Part model, mm, in its own coordinate system. A direction names the side the tool comes from. Give positions to 0.01 mm unless a question says otherwise; leave off trailing zeros. Order: outer loops, then holes, each group sorted by start corner. A loop starts at its lowest first (then second) coordinate and runs counter-clockwise, first axis right, second up. Notation, with made-up numbers: M 14.5,48 L 46.5,48 A33 ccw 46.5,80 Z; hole C 0.25,-4 d5. An arc over 180 degrees is marked long. Return JSON: item names as keys, results as strings.
from build123d import *

# Parameters (mm, degrees)
F1_DEPTH      = 10
F2_R          = 8
F3_T          = -1.5
F4_W          = 14.2378706528
F4_H          = 10
F5_DEPTH      = 50
F7_W          = 14.2378706528
F7_H          = 10
F8_DEPTH      = 50
F6_W          = 14.2378706528
F6_H          = 10
F9_DEPTH      = 50
F10_T         = 1.5
F10_T3_DEPTH  = 13
F10_T5_DEPTH  = 17.2378706528
F10_T7_DEPTH  = 17.2378706528
F10_T10_ANGLE = 72.000000001
F10_T12_ANGLE = 72.000000001
F10_T14_ANGLE = 72.000000001
F10_T16_ANGLE = 72.000000001
F10_T18_ANGLE = 72.000000001


# Not quite as in the source:
# - a shell that OpenCascade refuses in one call is made with other operations: the cavity is built on its own and cut out


with BuildPart() as f1:
    # F0 (on Top) → F1 (new body)
    with BuildSketch(Plane.XY):
        Polygon((20.9232433585, 6.7983738762), (0, 22), (-20.9232433585, 6.7983738762), (-12.9312755504, -17.7983738762), (12.9312755504, -17.7983738762), align=None)
    extrude(amount=F1_DEPTH)

    # F2
    f2_edges = [f1.edges().sort_by_distance(p)[0] for p in [
        (20.923243, 6.798374, 5),
        (0, 22, 5),
        (12.931276, -17.798374, 5),
        (-12.931276, -17.798374, 5),
        (-20.923243, 6.798374, 5),
    ]]
    fillet(f2_edges, radius=F2_R)

    # F3
    f3_openings = [f1.faces().sort_by_distance(p)[0] for p in [
        (0, 0, 0),
    ]]
    offset(amount=F3_T, openings=f3_openings)

    # F4 (on face) → F5 (join)
    with BuildSketch(Plane(origin=(16.9272594545, -5.5, 0), x_dir=(0.3090169944, 0.9510565163, 0), z_dir=(0.9510565163, -0.3090169944, 0))):
        with Locations((0, 5)):
            Rectangle(F4_W, F4_H)
    extrude(amount=F5_DEPTH)

    # F7 (on face) → F8 (join)
    with BuildSketch(Plane(origin=(10.4616216792, 14.3991869381, 0), x_dir=(-0.8090169944, 0.5877852523, 0), z_dir=(0.5877852523, 0.8090169944, 0))):
        with Locations((0, 5)):
            Rectangle(F7_W, F7_H)
    extrude(amount=F8_DEPTH)

    # F6 (on face) → F9 (join)
    with BuildSketch(Plane(origin=(-16.9272594545, -5.5, 0), x_dir=(0.3090169944, -0.9510565163, 0), z_dir=(-0.9510565163, -0.3090169944, 0))):
        with Locations((0, 5)):
            Rectangle(F6_W, F6_H)
    extrude(amount=F9_DEPTH)

    # F10: shell of thickness 1.5, made by hand


with BuildPart() as f10_core1:
    # F10_t2: copy of F1
    add(f1.part)

    # the walls: a layer under each face that stays
    f10_faces = [f10_core1.faces().sort_by_distance(p)[0] for p in [
        (0, 20.11145618, 5),
        (-10.4616216792, 14.3991869381, 5),
        (-19.1271314522, 6.2147817412, 5),
        (-11.8212173447, -16.2705098312, 5),
        (0, -17.7983738762, 5),
        (11.8212173447, -16.2705098312, 5),
        (38.5038003641, -19.9959346906, 5),
        (42.9035443596, -6.4549150281, 5),
        (19.1271314522, 6.2147817412, 5),
        (30.9155926475, 30.4402066006, 5),
        (19.3969133257, 38.8090169944, 5),
        (17.7005466777, 5.7512562497, 4.25),
        (10.9395394663, -15.0569843397, 4.25),
        (0, -16.2983738762, 4.25),
        (-10.9395394663, -15.0569843397, 4.25),
        (-17.7005466777, 5.7512562497, 4.25),
        (-9.5799438008, 13.1856614466, 4.25),
        (0, 18.61145618, 4.25),
        (0, 15.6565411519, 10),
        (-42.9035443596, -6.4549150281, 5),
        (-38.5038003641, -19.9959346906, 5),
        (0, 1.1565411519, 8.5),
    ]]
    thicken(f10_faces, amount=-F10_T, mode=Mode.SUBTRACT)

    # F10_s4 → F10_t3 (cut)
    with BuildSketch(Plane.XY.offset(-1.5)):
        Polygon((4.6989635422, 18.6045441687), (3.8206041399, 17.3700666434), (5.0341296315, 16.488388765), (5.9158075099, 17.7019142566), align=None)
        Polygon((-19.1460325548, 1.2801404241), (-17.7005466777, 1.7340353228), (-17.2370211862, 0.3074505484), (-18.6636059606, -0.1560749432), align=None)
        Polygon((-14.7370180496, -12.2894109339), (-13.3008026823, -11.8069843397), (-13.7643281739, -10.3803995652), (-15.1909129483, -10.8439250568), align=None)
        Polygon((14.7370180496, -12.2894109339), (13.3008026823, -11.8069843397), (13.7643281739, -10.3803995652), (15.1909129483, -10.8439250568), align=None)
        Polygon((19.1460325548, 1.2801404241), (18.6636059606, -0.1560749432), (17.2370211862, 0.3074505484), (17.7005466777, 1.7340353228), align=None)
        Polygon((16.2419133739, 10.2181002174), (15.3392834617, 9.0012562497), (14.1257579702, 9.8829341281), (15.0074358486, 11.0964596197), align=None)
    extrude(amount=F10_T3_DEPTH, mode=Mode.SUBTRACT)

    # F10_s6 → F10_t5 (cut)
    with BuildSketch(Plane.YZ.offset(-8.6189353264)):
        Polygon((-16.2833738762, 8.485), (-17.7983738762, 8.5), (-17.7983738762, 10), (-16.2983738762, 10), align=None)
    extrude(amount=F10_T5_DEPTH, mode=Mode.SUBTRACT)

    # F10_s8 → F10_t7 (cut)
    with BuildSketch(Plane(origin=(6.9728651525, 5.0660830753, 0), x_dir=(0, 0, 1), z_dir=(-0.8090169944, -0.5877852523, 0))):
        Polygon((8.485, 16.2833738762), (8.5, 17.7983738762), (10, 17.7983738762), (10, 16.2983738762), align=None)
    extrude(amount=F10_T7_DEPTH, mode=Mode.SUBTRACT)

    # F10_s9 → F10_t10 (revolve, cut)
    with BuildSketch(Plane(origin=(2.1998719977, 6.7705098312, 0), x_dir=(0, 0, 1), z_dir=(-0.3090169944, -0.9510565163, 0))):
        Polygon((8.485, -16.2833738762), (8.5, -17.7983738762), (10, -17.7983738762), (10, -16.2983738762), align=None)
    revolve(axis=Axis((11.5186793218, 3.7426457862, 8.5), (0, 0, 1)), revolution_arc=F10_T10_ANGLE, mode=Mode.SUBTRACT)

    # F10_s11 → F10_t12 (revolve, cut)
    with BuildSketch(Plane.YZ.offset(7.1189353264)):
        Polygon((-16.2833738762, 8.485), (-17.7983738762, 8.5), (-17.7983738762, 10), (-16.2983738762, 10), align=None)
    revolve(axis=Axis((7.1189353264, -9.7983738762, 8.5), (0, 0, 1)), revolution_arc=F10_T12_ANGLE, mode=Mode.SUBTRACT)

    # F10_s13 → F10_t14 (revolve, cut)
    with BuildSketch(Plane(origin=(2.1998719977, -6.7705098312, 0), x_dir=(0, 0, 1), z_dir=(-0.3090169944, 0.9510565163, 0))):
        Polygon((8.485, -16.2833738762), (8.5, -17.7983738762), (10, -17.7983738762), (10, -16.2983738762), align=None)
    revolve(axis=Axis((-7.1189353264, -9.7983738762, 8.5), (0, 0, 1)), revolution_arc=F10_T14_ANGLE, mode=Mode.SUBTRACT)

    # F10_s15 → F10_t16 (revolve, cut)
    with BuildSketch(Plane(origin=(-5.7593396609, -4.1844051969, 0), x_dir=(0, 0, 1), z_dir=(0.8090169944, 0.5877852523, 0))):
        Polygon((8.485, -16.2833738762), (8.5, -17.7983738762), (10, -17.7983738762), (10, -16.2983738762), align=None)
    revolve(axis=Axis((-11.5186793218, 3.7426457862, 8.5), (0, 0, 1)), revolution_arc=F10_T16_ANGLE, mode=Mode.SUBTRACT)

    # F10_s17 → F10_t18 (revolve, cut)
    with BuildSketch(Plane(origin=(-5.7593396609, 4.1844051969, 0), x_dir=(0, 0, 1), z_dir=(0.8090169944, -0.5877852523, 0))):
        Polygon((8.485, -16.2833738762), (8.5, -17.7983738762), (10, -17.7983738762), (10, -16.2983738762), align=None)
    revolve(axis=Axis((0, 12.11145618, 8.5), (0, 0, 1)), revolution_arc=F10_T18_ANGLE, mode=Mode.SUBTRACT)


with BuildPart() as f1_1:
    add(f1.part)

    # what is left inside the walls is the cavity
    f10_cavity = [f10_core1.part.solids().sort_by_distance(p)[0] for p in [
        (24.715414, 25.972877, 0.015),
        (39.99038, -17.427366, 0.015),
        (-39.99038, -17.427366, 0.015),
    ]]
    add(f10_cavity, mode=Mode.SUBTRACT)


solid = f1_1.part
Q1. Band-saw the part on B-B (z = 1.5). Give the number of separate pieces and of enclosed holes in the cut face, then the cut area to 3 significant figures.
Established:
{"separate pieces": "3", "enclosed holes": "0", "area": "575 mm²"}
Q2. Band-saw the part on D-D (y = 49). Give the cut face in (x, z).
Established:
{"outline": "M 26.8,0 L 28.66,0 L 28.66,8.5 L 42.55,8.5 L 42.55,0 L 44.4,0 L 44.4,10 L 26.8,10 Z"}
Q3. Band-saw the part on A-A (y = -20). Give the cut face in (x, z), then the cut area to 3 significant figures.
Established:
{"outline": "M -64.79,8.5 L -43.37,8.5 L -43.37,0 L -38.52,0 L -38.52,10 L -64.79,10 Z; M 38.52,0 L 43.37,0 L 43.37,8.5 L 64.79,8.5 L 64.79,10 L 38.52,10 Z", "area": "161 mm²"}
Q4. 3-axis set-ups, long thin cutter, end or side, ignore diameter. For faces 4 (the flat face through (-12, 12, 0)), 5 (the flat face through (42.571, -6.347, 4.93)), 6 (the flat face through (38.171, -19.888, 4.93)), 7 (the cylindrical face through (10.893, -15.09, 4.31)): which of +Z, -Z, +X, -X, +Y, -Y reach the whole face in a straight line?
Established:
{"face 4": "-Z, +X, -X, +Y, -Y", "face 5": "+Z, -Z, +X", "face 6": "+Z, -Z, -Y", "face 7": "-Z"}
Q5. Two-plate mould, pull along Y, no slides. Class faces 1 (the flat face through (-38.171, -19.888, 4.93)), 2 (the cylindrical face through (-19.1, 6.3, 5.1)), 3 (the flat face through (19.191, 38.526, 4.93)): +Y half, -Y half, draft (parallel to the pull), parting line (faces both ways), or undercut.
Established:
{"face 1": "-Y half", "face 2": "undercut", "face 3": "+Y half"}
Q6. Band-saw the part on C-C (x = 10.5). Give the cut face in (y, z), then the cut area to 3 significant figures.
Established:
{"outline": "M -17.05,0 L -15.35,0 L -15.35,8.5 L 24.01,8.5 L 24.01,0 L 26.56,0 L 26.56,10 L -17.05,10 Z", "area": "102 mm²"}
Q7. Probe line 1 along Y through (x, z) = (32, 2.5); line 2 along Y through (x, z) = (35.5, 5); line 3 along Y through (x, z) = (39.5, 6). List the from-to ranges inside material, lowest first.
Established:
{"line 1": "y = -17.88 to -16.31, -4.49 to -2.91, 31.93 to 34.48, 53.6 to 56.16", "line 2": "y = -19.02 to -17.44, -5.63 to -4.05, 36.75 to 39.3", "line 3": "y = -20.32 to -18.74, -6.93 to -5.35, 42.26 to 44.81"}
Q8. Pin check, flat tips, straight feed: pin 1 (3 mm diameter, centred on y = 5, z = 5, fed in from +X); pin 2 (1.5 mm diameter, centred on y = 19, z = 3, fed in from -X); pin 3 (4 mm diameter, centred on x = 42, z = 3.5, fed in from -Y). Stop position of each tip, or through.
Established:
{"pin 1": "stops at x = 19.52", "pin 2": "stops at x = -5.16", "pin 3": "stops at y = -21.78"}
